```python
from build123d import *

# Parameters (mm, degrees)
SKETCH2_R = 1.980736
FILLET2_R = 100


with BuildPart() as part:
    # Sketch1 → Cup (revolve)
    with BuildSketch(Plane(origin=(0, 0, 0), x_dir=(-1, 0, 0), z_dir=(0, 1, 0)), mode=Mode.PRIVATE) as cup_sk:
        Polygon((0, 3), (-27.6, 3), (-27.6, 0), (-29.573, 0), (-44.616104, 110.4), (-42.635368, 110.4), (-28.23035, 5), (0, 5), align=None)
    revolve(cup_sk.sketch.rotate(Axis((0, 0, -50), (0, 0, 1)), 180), axis=Axis((0, 0, -50), (0, 0, 1)))

    # Sketch2 → BeadRound (revolve)
    with BuildSketch(Plane(origin=(0, 0, 0), x_dir=(-1, 0, 0), z_dir=(0, 1, 0))):
        with Locations((-44.616104, 110.4)):
            Circle(SKETCH2_R)
    revolve(axis=Axis((0, 0, -50), (0, 0, 1)))

    # Fillet2
    fillet2_edges = [part.edges().sort_by_distance(p)[0] for p in [
        (0, -42.635368, 110.4),
    ]]
    fillet(fillet2_edges, radius=FILLET2_R)


solid = part.part
```
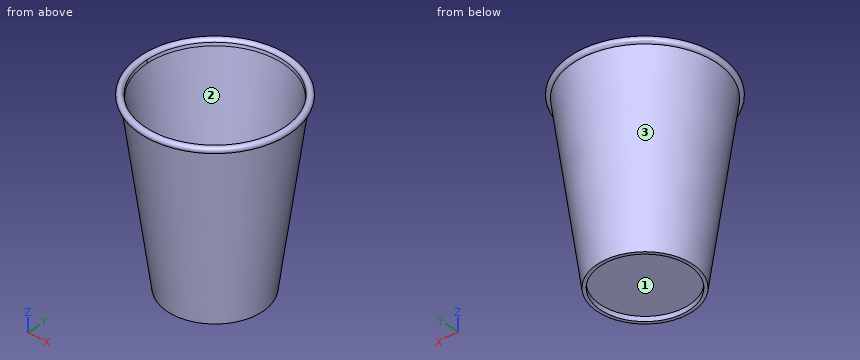
Model file for the job. Use its own axes, mm. Face numbers are marked on the shaded views. Round coordinates to 2 decimals unless told otherwise and drop trailing zeros. Loops run counter-clockwise (first coordinate to the right, second up) from the corner with the lowest first, then second, coordinate; pieces in that order, holes last. Notation, with made-up numbers: M -12.75,17 L 39.25,17 A32 cw 39.25,54 Z; hole C 8,-28.75 d6. An arc over 180 degrees is marked long. Put each result on its own line as item: value. Start each with the question number.
Item 1: Mould opens along X. For the marked faces 1, 2 and 3 say: released by +X, released by -X, zero draft, split by the parting line, or undercut.
Item 2: Drill centre lines: line 1 along Z through (x, y) = (11.5, -24); line 2 along Y through (x, z) = (31.5, 60); line 3 along Y through (x, z) = (-22, 102). Where is each one in solid material? Low to high.
Item 3: Cut at A-A (z = 70). List the corners of the cut face in (x, y), then the cut area to 3 significant figures.
Item 4: Drop flat-ended pins along their axis: P1, Ø1.5, axis at y = -21.5, z = 70, coming from the +X side; P2, Ø12, axis at y = -36, z = 92.5, coming from the +X side; P3, Ø3, axis at x = 27.5, z = 46.5, coming from the -Y side. Give the stop position or say it passes through.
Item 5: Cut at B-B (z = 25). List the corners of the cut face in (x, y).
Answer block:
1. face 1: undercut
1. face 2: undercut
1. face 3: split by the parting line
2. line 1: 3 to 5
2. line 2: -20.8 to -16.9, 16.9 to 20.8
2. line 3: -37.49 to -35.17, 35.17 to 37.49
3. outline: C 0,0 d78.22; hole C 0,0 d74.23
3. area: 478 mm2
4. P1: x = 33.17
4. P2: x = 29.76
4. P3: y = -24.8
5. outline: C 0,0 d65.96; hole C 0,0 d61.93
